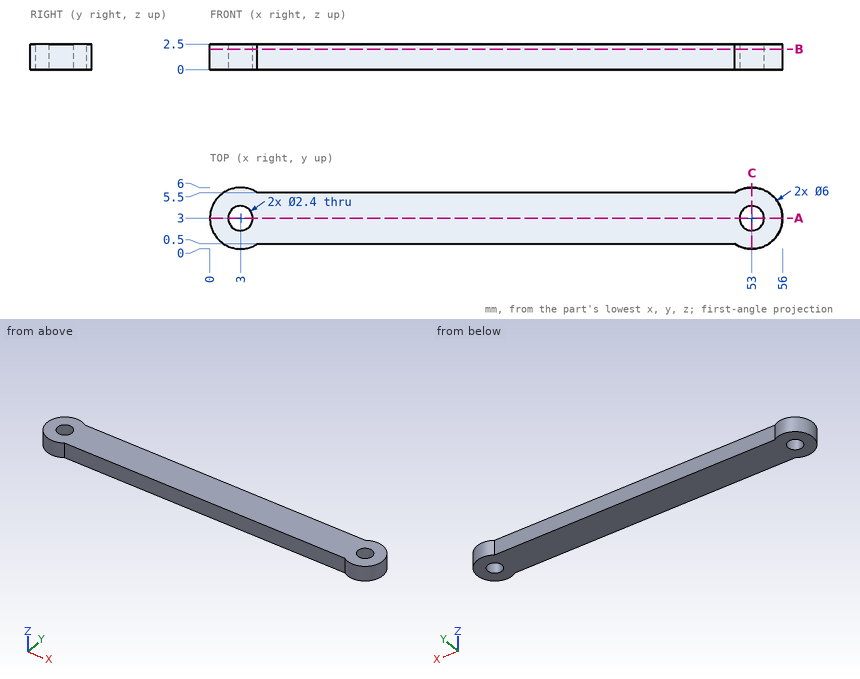
Source: three-view drawing plus pictorial views. Frame: mm from the lowest corner of the part. Round coordinates to 2 decimals unless told otherwise and drop trailing zeros. Write each loop counter-clockwise with the first axis right and the second up, starting at its lowest first coordinate (ties: lowest second). Pieces come first, ordered by that corner, then holes. Notation, with made-up numbers: (20.25, -29.75) -> (52.25, -29.75) arc R11 ccw to (52.25, -13.75) -> close; hole circle Ø6 at (32, 69.25). An arc over 180 degrees is marked (long way). Return JSON: item names as keys, results as strings.
Q1. Section A-A on y = 3. Return the cut outline in (x, z).
From the geometry:
{"outline": "(0, 0) -> (1.8, 0) -> (1.8, 2.5) -> (0, 2.5) -> close; (4.2, 0) -> (51.8, 0) -> (51.8, 2.5) -> (4.2, 2.5) -> close; (54.2, 0) -> (56, 0) -> (56, 2.5) -> (54.2, 2.5) -> close"}
Q2. Ray query, line 1 (X direction, y = 3.85, z = 1.4); line 2 (Y direction, x = 3, z = 1.45); line 3 (X direction, y = 3.7, z = 1.55). Return the intervals inside material, ascending.
From the geometry:
{"line 1": "0.12 to 2.15, 3.85 to 52.15, 53.85 to 55.88", "line 2": "0 to 1.8, 4.2 to 6", "line 3": "0.08 to 2.03, 3.97 to 52.03, 53.97 to 55.92"}
Q3. First-contact query: pin 1 Ø1.9 at (x, y) = (53, 3) entering from -Z; pin 2 Ø0.8 at (x, z) = (29.5, 1.5) entering from +Y. Flat tips, straight axial feed; report the tip coordinate or a pass-through.
From the geometry:
{"pin 1": "through", "pin 2": "y = 5.5"}
Q4. Section C-C on x = 53. Return the cut outline in (y, z).
From the geometry:
{"outline": "(0, 0) -> (1.8, 0) -> (1.8, 2.5) -> (0, 2.5) -> close; (4.2, 0) -> (6, 0) -> (6, 2.5) -> (4.2, 2.5) -> close"}
Q5. Section B-B on z = 2. Return the cut outline in (x, y), and give its area (3 significant figures).
From the geometry:
{"outline": "(4.66, 0.5) -> (51.34, 0.5) arc R3 ccw (long way) to (51.34, 5.5) -> (4.66, 5.5) arc R3 ccw (long way) to start; hole circle Ø2.4 at (3, 3); hole circle Ø2.4 at (53, 3)", "area": "271 mm2"}
